Read the model definition and answer for the solid it produces. Units are mm, in the model's axes. Face numbers are marked on the shaded views. Coordinates: 2 decimals unless noted, no trailing zeros. Write each loop counter-clockwise with the first axis right and the second up, starting at its lowest first coordinate (ties: lowest second). Pieces come first, ordered by that corner, then holes. Notation, with made-up numbers: (53.5, 74.5) - (57.5, 74.5) arc R29 ccw to (57.5, 95.5) - close; hole circle Ø8 at (-19, -11). An arc over 180 degrees is marked (long way). Use a Markdown table: item, result.
from build123d import *

# Parameters (mm, degrees)
F0_R     = 3.175
F1_DEPTH = 12.7
F2_R     = 38.1
F2_R_2   = 31.75
F3_DEPTH = 25.4


with BuildPart() as f1:
    # F0 (on Front) → F1 (new body)
    with BuildSketch(Plane.XZ):
        with BuildLine():
            Line((63.203057, 85.672887), (-57.446943, 85.672887))
            ThreePointArc((-57.446943, 85.672887), (-61.937071, 83.813015), (-63.796943, 79.322887))
            Line((-63.796943, 79.322887), (-63.796943, -41.327113))
            ThreePointArc((-63.796943, -41.327113), (-61.937071, -45.817241), (-57.446943, -47.677113))
            Line((-57.446943, -47.677113), (63.203057, -47.677113))
            ThreePointArc((63.203057, -47.677113), (67.693185, -45.817241), (69.553057, -41.327113))
            Line((69.553057, -41.327113), (69.553057, 79.322887))
            ThreePointArc((69.553057, 79.322887), (67.693185, 83.813015), (63.203057, 85.672887))
        make_face()
        with Locations((-57.446943, -41.327113)):
            Circle(F0_R, mode=Mode.SUBTRACT)
        with Locations((63.203057, -41.327113)):
            Circle(F0_R, mode=Mode.SUBTRACT)
        with Locations((-57.446943, 79.322887)):
            Circle(F0_R, mode=Mode.SUBTRACT)
        with Locations((63.203057, 79.322887)):
            Circle(F0_R, mode=Mode.SUBTRACT)
    extrude(amount=F1_DEPTH)

    # F2 (on face) → F3 (join)
    with BuildSketch(Plane.XZ.offset(12.7)):
        with Locations((2.878057, 18.997887)):
            Circle(F2_R)
        with Locations((2.878057, 18.997887)):
            Circle(F2_R_2, mode=Mode.SUBTRACT)
    extrude(amount=F3_DEPTH)


solid = f1.part
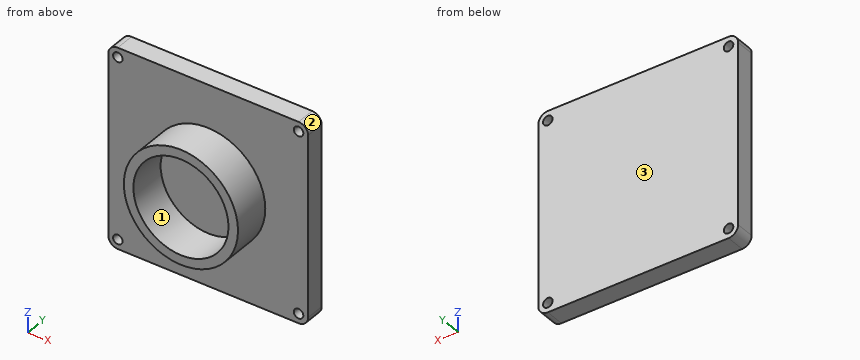
(1) The mould has two halves that part along X. Classify the marked faces 1, 2 and 3: pulls with the +X half, pulls with the -X half, needs draft (parallel to the pull), parting line crosses it, or undercut.
Report:
| item | result |
|---|---|
| face 1 | undercut |
| face 2 | pulls with the +X half |
| face 3 | needs draft |
(2) A cutting plane is placed at A-A, the plane z = -8. Write down the section's boundary in (x, y), and give its area (3 significant figures).
Report:
| item | result |
|---|---|
| outline | (-63.8, -12.7) - (-24.01, -12.7) - (-24.01, -38.1) - (-13.83, -38.1) - (-13.83, -12.7) - (19.59, -12.7) - (19.59, -38.1) - (29.76, -38.1) - (29.76, -12.7) - (69.55, -12.7) - (69.55, 0) - (-63.8, 0) - close |
| area | 2,210 mm² |
(3) A cutting plane is placed at B-B, the plane x = -3.5. Write down the section's boundary in (y, z), and give its area (3 significant figures).
Report:
| item | result |
|---|---|
| outline | (-38.1, -18.56) - (-12.7, -18.56) - (-12.7, -47.68) - (0, -47.68) - (0, 85.67) - (-12.7, 85.67) - (-12.7, 56.56) - (-38.1, 56.56) - (-38.1, 50.1) - (-12.7, 50.1) - (-12.7, -12.1) - (-38.1, -12.1) - close |
| area | 2,020 mm² |
(4) A cutting plane is placed at D-D, the plane x = 56. Write down the section's boundary in (y, z), and give its area (3 significant figures).
Report:
| item | result |
|---|---|
| outline | (-12.7, -47.68) - (0, -47.68) - (0, 85.67) - (-12.7, 85.67) - close |
| area | 1,690 mm² |
(5) Straight lines are drawn through the part: L1, parallel to Z at x = 2.5, y = -26.5; L2, parallel to Y at x = 4.5, z = 32.5; L3, parallel to Z at x = -3, y = -13. For each, find the intervals that lie inside material, in ascending order.
Report:
| item | result |
|---|---|
| L1 | z = -19.1 to -12.75, 50.75 to 57.1 |
| L2 | y = -12.7 to 0 |
| L3 | z = -18.65 to -12.2, 50.2 to 56.64 |
(6) A cutting plane is placed at C-C, the plane y = -24. Write down the section's boundary in (x, z), and give its area (3 significant figures).
Report:
| item | result |
|---|---|
| outline | circle Ø76.2 at (2.88, 19); hole circle Ø63.5 at (2.88, 19) |
| area | 1,390 mm² |
(7) Each of these flat-tipped pins is pushed along its axis until it touches: P1, Ø3, axis at x = 22, y = -25.5, coming from the +Z side; P2, Ø7.5, axis at x = -57.45, z = -41.33, coming from the -Y side; P3, Ø3, axis at y = -32.5, z = 10.5, coming from the -X side. Where does it stop, or does it pass through?
Report:
| item | result |
|---|---|
| P1 | stops at z = 52.78 |
| P2 | stops at y = -12.7 |
| P3 | stops at x = -34.57 |
